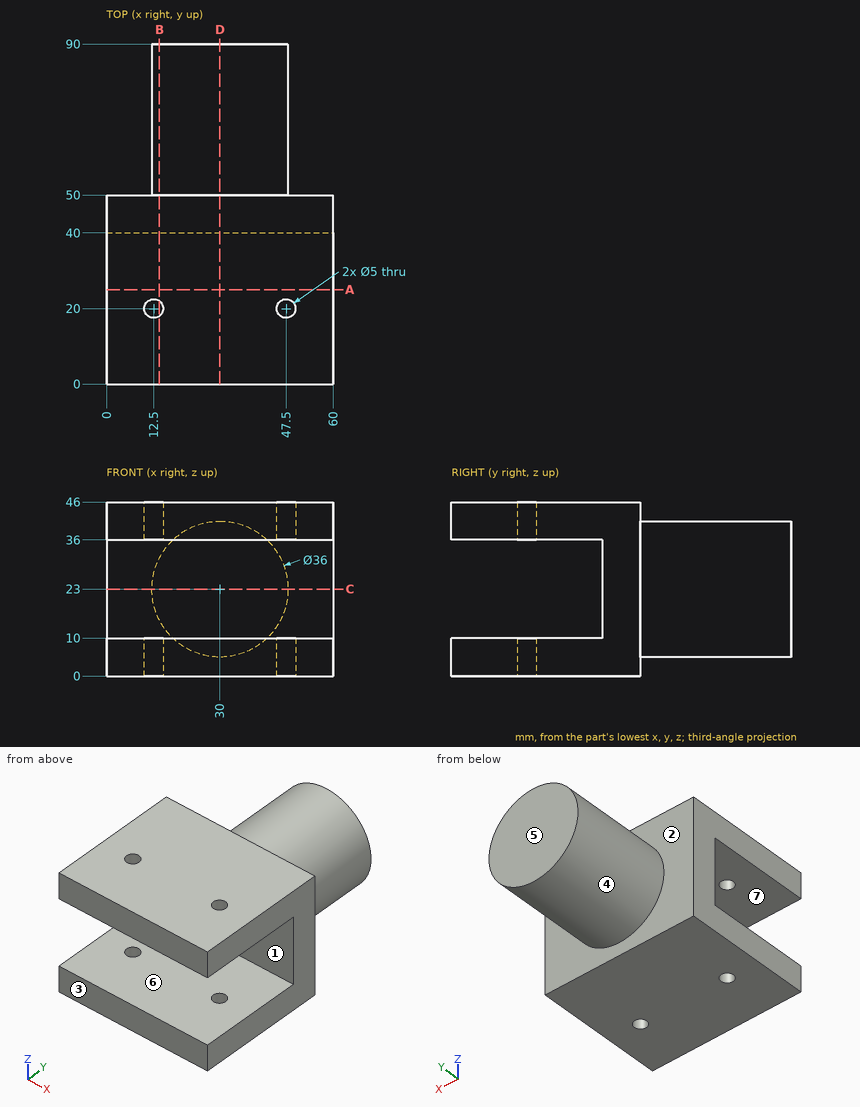
Answer from the drawing. Dimensions are ordinates in mm from the lowest x, y and z of the part. A direction names the side the tool comes from. Give positions to 0.01 mm unless a question says otherwise; leave off trailing zeros. Loops run counter-clockwise (first coordinate to the right, second up) from the corner with the lowest first, then second, coordinate; pieces in that order, holes last. Notation, with made-up numbers: (85.25, -2.75) -> (116.25, -2.75) arc R30 cw to (116.25, 24.25) -> close; hole circle Ø6 at (11, -28). An arc over 180 degrees is marked (long way). Answer as CSV lines item,"result".
Item 1: Find section D-D on x = 30. Give the vertices of the cut face in (y, z).
Returned:
outline,"(0, 0) -> (50, 0) -> (50, 5) -> (90, 5) -> (90, 41) -> (50, 41) -> (50, 46) -> (0, 46) -> (0, 36) -> (40, 36) -> (40, 10) -> (0, 10) -> close"
Item 2: Determine the mould class of the marked faces 4, 5, 6 and 7 for opening direction Z: +Z half, -Z half, draft (parallel to the pull), parting line (faces both ways), or undercut.
Returned:
face 4,"parting line"
face 5,"draft"
face 6,"undercut"
face 7,"undercut"
Item 3: Each of these flat-tipped pins is pushed along its axis until it touches: pin 1 (8 mm diameter, centred on x = 45, y = 58, fed in from +Z); pin 2 (1 mm diameter, centred on x = 46, y = 20, fed in from +Z); pin 3 (2 mm diameter, centred on x = 37, z = 21, fed in from -Y). Where does it stop, or does it pass through?
Returned:
pin 1,"stops at z = 37.25"
pin 2,"passes through"
pin 3,"stops at y = 40"
Item 4: Find section A-A on y = 25. Give the vertices of the cut face in (x, z), plus the area to 3 significant figures.
Returned:
outline,"(0, 0) -> (60, 0) -> (60, 10) -> (0, 10) -> close; (0, 36) -> (60, 36) -> (60, 46) -> (0, 46) -> close"
area,"1,200 mm²"
Item 5: Consider line 1 (Z direction, x = 57.5, y = 22); line 2 (Y direction, x = 47.5, z = 7); line 3 (X direction, y = 22, z = 9). Determine where each line is inside the solid, lowest interval first. Write a range as [from, to].
Returned:
line 1,"z = [0, 10], [36, 46]"
line 2,"y = [0, 17.5], [22.5, 50]"
line 3,"x = [0, 11], [14, 46], [49, 60]"
Item 6: Find section C-C on z = 23. Give the vertices of the cut face in (x, y), plus the area to 3 significant figures.
Returned:
outline,"(0, 40) -> (60, 40) -> (60, 50) -> (48, 50) -> (48, 90) -> (12, 90) -> (12, 50) -> (0, 50) -> close"
area,"2,040 mm²"
Item 7: Find section B-B on x = 14. Give the vertices of the cut face in (y, z), plus the area to 3 significant figures.
Returned:
outline,"(0, 0) -> (18, 0) -> (18, 10) -> (0, 10) -> close; (0, 36) -> (18, 36) -> (18, 46) -> (0, 46) -> close; (22, 0) -> (50, 0) -> (50, 14.75) -> (90, 14.75) -> (90, 31.25) -> (50, 31.25) -> (50, 46) -> (22, 46) -> (22, 36) -> (40, 36) -> (40, 10) -> (22, 10) -> close"
area,"1,840 mm²"
Item 8: For the marked faces 1, 2 and 3, determine the directions among +Z, -Z, +X, -X, +Y, -Y from which every point of the face is accessible in a straight line to the end or side of a thin tool.
Returned:
face 1,"+X, -X, -Y"
face 2,"+Y"
face 3,"+Z, -Z, +X, -X, -Y"
